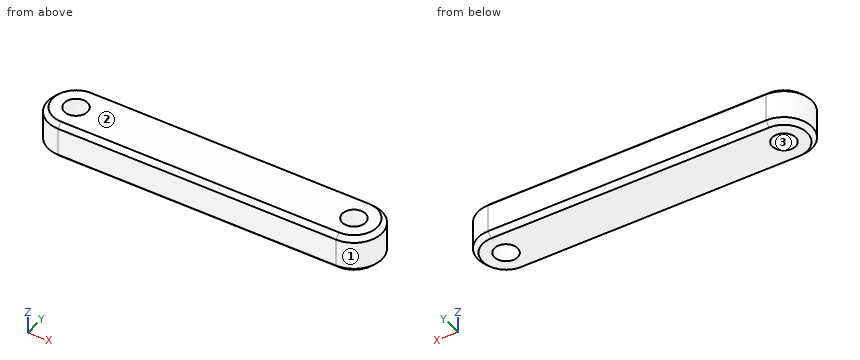
```python
from build123d import *

# Parameters (mm, degrees)
CROQUIS1_R              = 1.25
SALIENTE_EXTRUIR1_DEPTH = 4
CHAFL_N1_SIZE           = 0.5


with BuildPart() as part:
    # Croquis1 → Saliente-Extruir1 (new body)
    with BuildSketch(Plane.XY):
        with BuildLine():
            Line((0, 3), (30, 3))
            ThreePointArc((30, 3), (33, 0), (30, -3))
            Line((30, -3), (0, -3))
            ThreePointArc((0, -3), (-3, 0), (0, 3))
        make_face()
        with Locations((30, 0)):
            Circle(CROQUIS1_R, mode=Mode.SUBTRACT)
        Circle(CROQUIS1_R, mode=Mode.SUBTRACT)
    extrude(amount=SALIENTE_EXTRUIR1_DEPTH)

    # Chaflán1
    chafl_n1_edges = [part.edges().sort_by_distance(p)[0] for p in [
        (33, 0, 4),
        (15, 3, 4),
        (-3, 0, 4),
        (15, 3, 0),
        (33, 0, 0),
        (15, -3, 0),
        (-3, 0, 0),
        (15, -3, 4),
    ]]
    chamfer(chafl_n1_edges, length=CHAFL_N1_SIZE)


solid = part.part
```
Verification items for the finished model (mm, model axes). Face numbers are marked on the shaded views. Round coordinates to 2 decimals unless told otherwise and drop trailing zeros. Write each loop counter-clockwise with the first axis right and the second up, starting at its lowest first coordinate (ties: lowest second). Pieces come first, ordered by that corner, then holes. Notation, with made-up numbers: (3.25, 58) - (61.25, 58) arc R19 ccw to (61.25, 86) - close; hole circle Ø8 at (1.5, -18). An arc over 180 degrees is marked (long way). Answer as a JSON object with one key per item and string values. Group by question number.
Q1. Section check A-A, the plane y = 0. Enter the section's corners in (x, z).
Q2. Section check B-B, the plane x = 6. Enter the section's corners in (y, z).
Q3. Mould release check, pull along X, two halves, no side actions. Record for the marked faces 1, 2 and 3: released by +X, released by -X, zero draft, split by the parting line, or undercut.
Q4. Section check C-C, the plane z = 1.9. Enter the section's corners in (x, y), plus the area to 3 significant figures.
Q5. Thickness scan on line 1 (X direction, y = 0.2, z = 2.4); line 2 (Y direction, x = 0, z = 2.1); line 3 (Y direction, x = 1, z = 3.4). Record the ranges inside material, lowest first.
Found:
{
 "1": {"outline": "(-3, 0.5) - (-2.5, 0) - (-1.25, 0) - (-1.25, 4) - (-2.5, 4) - (-3, 3.5) - close; (1.25, 0) - (28.75, 0) - (28.75, 4) - (1.25, 4) - close; (31.25, 0) - (32.5, 0) - (33, 0.5) - (33, 3.5) - (32.5, 4) - (31.25, 4) - close"},
 "2": {"outline": "(-3, 0.5) - (-2.5, 0) - (2.5, 0) - (3, 0.5) - (3, 3.5) - (2.5, 4) - (-2.5, 4) - (-3, 3.5) - close"},
 "3": {"face 1": "released by +X", "face 2": "zero draft", "face 3": "undercut"},
 "4": {"outline": "(0, -3) - (30, -3) arc R3 ccw to (30, 3) - (0, 3) arc R3 ccw to start; hole circle Ø2.5 at (0, 0); hole circle Ø2.5 at (30, 0)", "area": "198 mm^2"},
 "5": {"line 1": "x = -2.99 to -1.23, 1.23 to 28.77, 31.23 to 32.99", "line 2": "y = -3 to -1.25, 1.25 to 3", "line 3": "y = -3 to -0.75, 0.75 to 3"}
}
